Can you work these out from the model? Positions are in its coordinate system, mm. Face numbers are marked on the shaded views. A direction names the side the tool comes from. Coordinates: 2 decimals unless noted, no trailing zeros. Loops run counter-clockwise (first coordinate to the right, second up) from the corner with the lowest first, then second, coordinate; pieces in that order, holes last. Notation, with made-up numbers: M 24,79.5 L 71,79.5 A21 cw 71,84.5 Z; hole C 49.25,67 d3. An arc over 180 degrees is marked long. Answer as a JSON object with one key per item and string values. Group by question number.
Item 1: If I drill on line 1 (Y direction, x = 0.5, z = 1.7); line 2 (Y direction, x = 1, z = 2.95); line 3 (Y direction, x = -11, z = 4.1), over which ranges is the centre line in solid material (lowest first)?
Item 2: Suppose I cut it at C-C (y = 12). Write out the boundary of the cut face in (x, z).
Item 3: Suppose I cut it at A-A (y = 0). Write out the boundary of the cut face in (x, z), then the cut area to 3 significant figures.
Item 4: Which directions (+Z, -Z, +X, -X, +Y, -Y) give clear straight access to the entire face, cutting with the end or side of a thin tool? Please do the marked faces 4 and 5.
Item 5: Suppose I cut it at B-B (z = 5.4). Count the separate pieces of the cut face and the enclosed holes in it, then the cut area to 3 significant figures.
Item 6: I'm going to push flat-ended pins straight in: pin 1 Ø1 at (x, z) = (-1, 4) entering from +Y; pin 2 Ø1.3 at (x, y) = (-0.5, -8.5) entering from +Z. Where does each tip first touch, or does it pass through?
Item 7: We'd pull the mould along Y, two halves only. Please class the marked faces 1, 2 and 3: +Y half, -Y half, draft (parallel to the pull), parting line (faces both ways), or undercut.
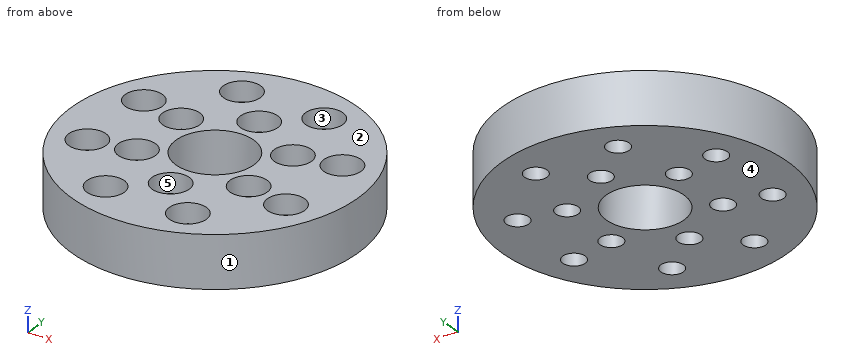
```python
from build123d import *

# Parameters (mm, degrees)
SKETCH_1_R                = 16.5
SKETCH_1_R_2              = 4.5
EXTRUDE_1_DEPTH           = 6
HOLE_WIZARD_1_D           = 2.6
HOLE_WIZARD_1_CBORE_D     = 4.3
HOLE_WIZARD_1_CBORE_DEPTH = 2.3
PATTERN_CIRCULAR_1_COUNT  = 6
HOLE_WIZARD_2_D           = 2.6
HOLE_WIZARD_2_CBORE_D     = 4.3
HOLE_WIZARD_2_CBORE_DEPTH = 2.3
PATTERN_CIRCULAR_2_COUNT  = 8


with BuildPart() as part:
    # Sketch 1 → Extrude 1 (new body)
    with BuildSketch(Plane.XY):
        Circle(SKETCH_1_R)
        Circle(SKETCH_1_R_2, mode=Mode.SUBTRACT)
    extrude(amount=EXTRUDE_1_DEPTH)

    # Hole Wizard 1 (through all)
    with Locations(Plane.XY.offset(6)):
        with Locations((0, 7.5)):
            hole_wizard_1 = CounterBoreHole(HOLE_WIZARD_1_D / 2, HOLE_WIZARD_1_CBORE_D / 2, HOLE_WIZARD_1_CBORE_DEPTH)

    # Pattern Circular 1: Hole Wizard 1 ×6 about axis
    pattern_circular_1_axis = Axis((0, 0, 0), (0, 0, 1))
    for i in range(1, PATTERN_CIRCULAR_1_COUNT):
        add(hole_wizard_1.rotate(pattern_circular_1_axis, i * 360 / PATTERN_CIRCULAR_1_COUNT), mode=Mode.SUBTRACT)

    # Hole Wizard 2 (through all)
    with Locations(Plane.XY.offset(6)):
        with Locations((-4.783542905, 11.548494156)):
            hole_wizard_2 = CounterBoreHole(HOLE_WIZARD_2_D / 2, HOLE_WIZARD_2_CBORE_D / 2, HOLE_WIZARD_2_CBORE_DEPTH)

    # Pattern Circular 2: Hole Wizard 2 ×8 about axis
    pattern_circular_2_axis = Axis((0, 0, 0), (0, 0, 1))
    for i in range(1, PATTERN_CIRCULAR_2_COUNT):
        add(hole_wizard_2.rotate(pattern_circular_2_axis, i * 360 / PATTERN_CIRCULAR_2_COUNT), mode=Mode.SUBTRACT)


solid = part.part
```
From the geometry:
{
 "1": {"line 1": "-16.49 to -8.7, -6.3 to -4.47, 4.47 to 6.3, 8.7 to 16.49", "line 2": "-16.47 to -8.33, -6.67 to -4.39, 4.39 to 6.67, 8.33 to 16.47", "line 3": "-12.3 to -6.86, -2.7 to 2.7, 6.86 to 12.3"},
 "2": {"outline": "M -11.32,0 L -6,0 L -6,3.7 L -6.89,3.7 L -6.89,6 L -11.32,6 Z; M -3.56,0 L 3.56,0 L 3.56,3.7 L 2.68,3.7 L 2.68,6 L -2.68,6 L -2.68,3.7 L -3.56,3.7 Z; M 6,0 L 11.32,0 L 11.32,6 L 6.89,6 L 6.89,3.7 L 6,3.7 Z"},
 "3": {"outline": "M -16.5,0 L -4.5,0 L -4.5,6 L -16.5,6 Z; M 4.5,0 L 16.5,0 L 16.5,6 L 4.5,6 Z", "area": "144 mm2"},
 "4": {"face 4": "-Z, +X, -X, +Y, -Y", "face 5": "+Z"},
 "5": {"separate pieces": "1", "enclosed holes": "15", "area": "588 mm2"},
 "6": {"pin 1": "y = 16.49", "pin 2": "z = 3.7"},
 "7": {"face 1": "parting line", "face 2": "draft", "face 3": "undercut"}
}
